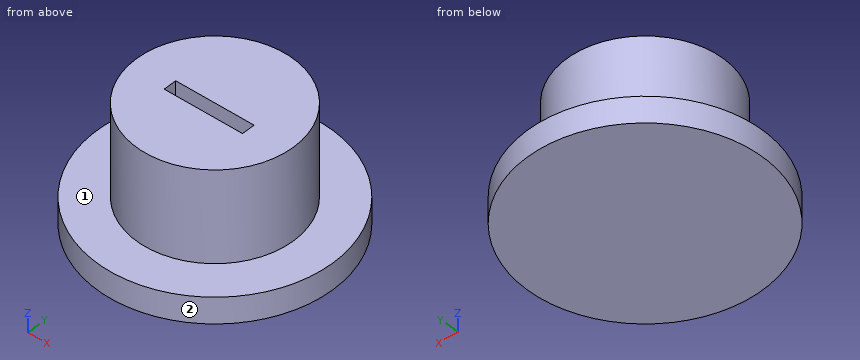
from build123d import *

# Parameters (mm, degrees)
F0_R     = 4.5
F1_DEPTH = 1
F2_R     = 3
F3_DEPTH = 3.5
F4_W     = 3
F4_H     = 0.75
F5_DEPTH = 2
F6_W     = 3
F6_H     = 0.25
F7_DEPTH = 1.2


with BuildPart() as f1:
    # F0 (on Top) → F1 (new body)
    with BuildSketch(Plane.XY):
        Circle(F0_R)
    extrude(amount=F1_DEPTH)

    # F2 (on face) → F3 (join)
    with BuildSketch(Plane.XY.offset(1)):
        Circle(F2_R)
    extrude(amount=F3_DEPTH)

    # F4 (on face) → F5 (cut)
    with BuildSketch(Plane.XY.offset(4.5)):
        with Locations((0, -0.125)):
            Rectangle(F4_W, F4_H)
    extrude(amount=-F5_DEPTH, mode=Mode.SUBTRACT)

    # F6 (on face) → F7 (join)
    with BuildSketch(Plane.XY.offset(4.5)):
        with Locations((0, 0.125)):
            Rectangle(F6_W, F6_H)
    extrude(amount=-F7_DEPTH)


solid = f1.part
Geometry check sheet. Reference: the model listing, model coordinates, mm. Face numbers are marked on the shaded views. A direction names the side the tool comes from. Give positions to 0.01 mm unless a question says otherwise; leave off trailing zeros. Write each loop counter-clockwise with the first axis right and the second up, starting at its lowest first coordinate (ties: lowest second). Pieces come first, ordered by that corner, then holes. Notation, with made-up numbers: M 12,36.5 L 65,36.5 A9 ccw 65,47.5 Z; hole C 18.25,70.5 d3. An arc over 180 degrees is marked long. Answer as CSV lines item,"result". Start each with the question number.
Q1. Section check A-A, the plane x = 0. Record the cut outline in (y, z), then the cut area to 3 significant figures.
Q2. Tool access check on the marked faces 1 and 2. Record the directions out of +Z, -Z, +X, -X, +Y, -Y that give a thin tool (end or side, any length) a straight path to the whole face; none if there is none.
Q3. Section check B-B, the plane y = -2.75. Record the cut outline in (x, z), then the cut area to 3 significant figures.
Q4. Material ranges on L1, parallel to Z at x = -4, y = 1.5; L2, parallel to Y at x = 0, z = 2.15; L3, parallel to Y at x = 0.75, z = 2.85, recorded low to high.
Q5. Go/stop test with flat-tipped pins: pin 1 (2 mm diameter, centred on y = -3, z = 3.5, fed in from +X); pin 2 (0.8 mm diameter, centred on y = 0, z = 4, fed in from +X); pin 3 (2 mm diameter, centred on x = -0.5, z = 4, fed in from +Y). Record where each tip stops, or that it passes through.
Q6. Section check D-D, the plane x = 1.25. Record the cut outline in (y, z).
Q7. Section check C-C, the plane z = 1.65. Record the cut outline in (x, y), then the cut area to 3 significant figures.
Geometry says:
1,outline,"M -4.5,0 L 4.5,0 L 4.5,1 L 3,1 L 3,4.5 L 0,4.5 L 0,3.3 L 0.25,3.3 L 0.25,2.5 L -0.5,2.5 L -0.5,4.5 L -3,4.5 L -3,1 L -4.5,1 Z"
1,area,"28.8 mm^2"
2,face 1,"+Z"
2,face 2,"+Z, -Z"
3,outline,"M -3.56,0 L 3.56,0 L 3.56,1 L 1.2,1 L 1.2,4.5 L -1.2,4.5 L -1.2,1 L -3.56,1 Z"
3,area,"15.5 mm^2"
4,L1,"0 to 1"
4,L2,"-3 to 3"
4,L3,"-2.9 to -0.5, 0.25 to 2.9"
5,pin 1,"x = 2.24"
5,pin 2,"x = 3"
5,pin 3,"y = 3"
6,outline,"M -4.32,0 L 4.32,0 L 4.32,1 L 2.73,1 L 2.73,4.5 L 0,4.5 L 0,3.3 L 0.25,3.3 L 0.25,2.5 L -0.5,2.5 L -0.5,4.5 L -2.73,4.5 L -2.73,1 L -4.32,1 Z"
7,outline,"C 0,0 d6"
7,area,"28.3 mm^2"
